Work out the finished part from the listing and answer in its coordinate system (mm). Face numbers are marked on the shaded views. Give positions to 0.01 mm unless a question says otherwise; leave off trailing zeros. Write each loop counter-clockwise with the first axis right and the second up, starting at its lowest first coordinate (ties: lowest second). Pieces come first, ordered by that corner, then holes.
1) Find section C-C (x = 4.25). Determine the outline of the cut face in (y, z), plus the area to 3 significant figures.
2) Determine the mould class of the marked faces 1, 2 and 3 for opening direction X: pulls with the +X half, pulls with the -X half, needs draft (parallel to the pull), parting line crosses it, or undercut.
3) Find section B-B (y = 0). Determine the outline of the cut face in (x, z), plus the area to 3 significant figures.
4) Straight lines are drawn through the part: probe 1 along X at (y, z) = (0.3, -0.3); probe 2 along Y at (x, z) = (5, 0.05); probe 3 along Y at (x, z) = (5.75, 0.9). For each, find the intervals that lie inside material, in ascending order.
5) Given pin 1 Ø0.6 at (y, z) = (0, -1) entering from -X; pin 2 Ø1.5 at (y, z) = (-1, 1) entering from +X; pin 3 Ø2 at (x, z) = (5, -1) entering from -Y, each flat-ended and moving along its own axis, determine where each tip first touches the part or whether it passes through.
6) Find section A-A (z = 0). Determine the outline of the cut face in (x, y).
Autodesk Inventor part; units mm, degrees
ref_plane "Work Plane1" through (33.575, 0, 0) normal (0, 0, -1) x (1, 0, 0)
ref_plane "YZ Plane" through (0, 0, 0) normal (1, 0, 0) x (0, 1, 0)
ref_plane "XZ Plane" through (0, 0, 0) normal (0, 1, 0) x (-1, 0, 0)
sketch "Sketch1" plane through (0, 0, 0) normal (0, 0, 1) x (1, 0, 0)
  line L0 (0, 0) -> (8, 0)
  line L1 (8, 0) -> (8, 1)
  line L2 (8, 1) -> (2, 1)
  line L3 (2, 1) -> (1.7546, 0.7546)
  line L4 (1.7546, 0.7546) -> (1.4454, 0.7546)
  line L5 (1.4454, 0.7546) -> (0.45, 1.75)
  line L6 (0.45, 1.75) -> (0, 1.75)
  line L7 (0, 1.75) -> (0, 0)
  line L8 (2, 1) -> (1.2, 1) construction
  line L9 (-1.6, 0) -> (9.6, 0)
  line L10 (0, 2.1) -> (0, -0.35)
  dimension "d0" = 8
  dimension "d1" = 45
  dimension "d2" = 0.2454
  dimension "d3" = 6
  dimension "d4" = 1.2
  dimension "d5" = 1.5092
  dimension "d6" = 2
  dimension "d7" = 3.5
revolve "Body" add sketch "Sketch1" angle 360 about axis through (0, 0, 0) along (1, 0, 0)
sketch "Sketch2" plane through (0, 0, 0) normal (-1, 0, 0) x (0, 0, 1)
  line L0 (1.75, -0.35) -> (-1.75, -0.35)
  line L1 (-1.75, -0.35) -> (-1.75, 0.35)
  line L2 (-1.75, 0.35) -> (1.75, 0.35)
  line L3 (1.75, 0.35) -> (1.75, -0.35)
  line L4 (0, 0.35) -> (0, -0.35) construction
  line L5 (-1.75, 0) -> (1.75, 0) construction
  line L6 (0, 1.75) -> (0, 0)
  dimension "d15" = 0.7
  dimension "d16" = 3.5
extrude "Slot" cut sketch "Sketch2" against normal blind 0.4
thread "Thread"
chamfer "Chamfer1" distance 0.2454 distance2 0.1227 1 edges at (8, -1, 0) measured on face at (8, -0.0858, 0.7069)
ref_plane "Work Plane1" through (33.575, 0, 0) normal (0, 0, -1) x (1, 0, 0)
equation "\"d0\" = NLG"
equation "\"d1\" = 0.5 * SEWI"
equation "\"d2\" = GAL"
equation "\"d3\" = GEL"
equation "\"d4\" = KOH"
equation "\"d5\" = BDM"
equation "\"d6\" = GD"
equation "\"d7\" = KOD"
equation "\"d15\" = SBR"
equation "\"d16\" = KOD"
equation "\"d8\" = STI"
equation "\"d10\" = GEL"
equation "\"d12\" = -0.5 * SPD + 0.5 * GD"
equation "\"d13\" = 0.5 * GAL"
equation "\"NLG\" = 8"
equation "\"GAL\" = 0.61345 * PTC"
equation "\"GEL\" = 6"
equation "\"KOH\" = 1.2"
equation "\"KOD\" = 3.5"
equation "\"SEWI\" = 90deg"
equation "\"BDM\" = NND - 1.2269 * PTC"
equation "\"GD\" = NND"
equation "\"SBR\" = 0.7"
equation "\"STI\" = 0.4"
equation "\"SPD\" = NND - 1.2269 * PTC"
equation "\"GUL\" = 0.61345 * PTC"
equation "\"PTC\" = 0.4"
equation "\"EPV\" = 2.2"
equation "\"THREADDIA\" = 2"
equation "\"TOA\" = 30deg"
equation "\"RR\" = 0.2"
equation "\"NND\" = 2"
equation "\"GD1\" = THREADDIA - 1.2269 * PTC"
properties part number "AS 1427 - M2 x 8(8)" material "Steel, Mild"
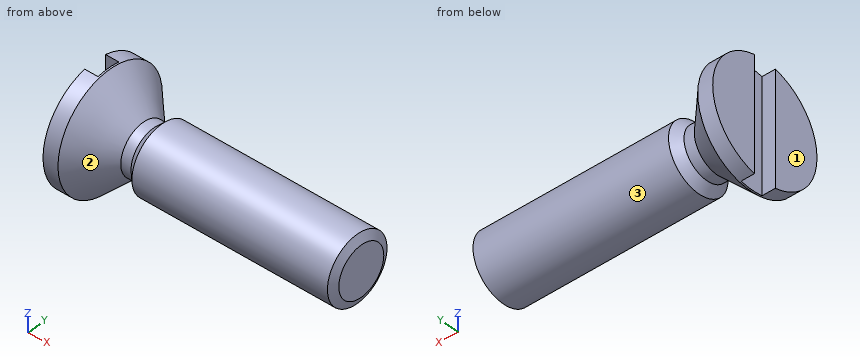
Results:
1. outline: circle Ø2 at (0, 0)
1. area: 3.14 mm2
2. face 1: pulls with the -X half
2. face 2: undercut
2. face 3: needs draft
3. outline: (0.4, -1.75) - (0.45, -1.75) - (1.45, -0.75) - (1.75, -0.75) - (2, -1) - (7.88, -1) - (8, -0.75) - (8, 0.75) - (7.88, 1) - (2, 1) - (1.75, 0.75) - (1.45, 0.75) - (0.45, 1.75) - (0.4, 1.75) - close
3. area: 15.5 mm2
4. probe 1: x = 0.4 to 8
4. probe 2: y = -1 to 1
4. probe 3: y = -0.44 to 0.44
5. pin 1: stops at x = 0.4
5. pin 2: stops at x = 8
5. pin 3: stops at y = -1
6. outline: (0, -1.75) - (0.45, -1.75) - (1.45, -0.75) - (1.75, -0.75) - (2, -1) - (7.88, -1) - (8, -0.75) - (8, 0.75) - (7.88, 1) - (2, 1) - (1.75, 0.75) - (1.45, 0.75) - (0.45, 1.75) - (0, 1.75) - (0, 0.35) - (0.4, 0.35) - (0.4, -0.35) - (0, -0.35) - close
